Input: part model. Units: mm. Frame: model coordinates. A direction names the side the tool comes from. Round coordinates to 2 decimals unless told otherwise and drop trailing zeros. Loops run counter-clockwise (first coordinate to the right, second up) from the corner with the lowest first, then second, coordinate; pieces in that order, holes last. Notation, with made-up numbers: (77.25, 69.5) -> (85.25, 69.5) arc R29 ccw to (85.25, 89.5) -> close; hole circle Ø10 at (25.5, -8.5). An arc over 180 degrees is marked (long way). Answer as a JSON object with one key per item and string values. Group by question number.
Item 1: Material intervals for line 1 (Y direction, x = 60, z = 59.5); line 2 (X direction, y = 62, z = 2); line 3 (Z direction, x = 28.5, y = 12.5), sorted ascending. Write a range as [from, to].
Item 2: Section query A-A on x = 0. Return loops of the section in (y, z).
Item 3: Draft query along Y for faces 1 (the flat face through (75.115, 1, -4)), 2 (the flat face through (-65, 71.785, 51)), 3 (the flat face through (65, -60.993, 51)). Return one class per face: released by +Y, released by -Y, zero draft, split by the parting line, or undercut.
Item 4: Section query D-D on x = 63.5. Return loops of the section in (y, z).
Item 5: Set-up query: faces 4 (the flat face through (-65, -71.785, 51)), 5 (the flat face through (70.377, 66, 51)), 6 (the flat face through (-59.117, -66, 51)), 7 (the flat face through (-70.377, -66, 51)), 8 (the cylindrical face through (-0.47, 21.17, -4.44)). Return all of +Z, -Z, +X, -X, +Y, -Y with unobstructed straight access to the full face (end or side cutting, diameter ignored); none if empty.
Item 6: Section query C-C on y = 17. Return loops of the section in (x, z), and give its area (3 significant figures).
Item 7: Section query B-B on z = 69. Return loops of the section in (x, y), and give its area (3 significant figures).
Item 8: Pin query (flat end, axial travel): pin 1 (12 mm diameter, centred on y = -68, z = 36, fed in from +X); pin 2 (8.5 mm diameter, centred on y = 65, z = 37, fed in from -X); pin 3 (2 mm diameter, centred on y = -58, z = 59, fed in from +X); pin 4 (5.5 mm diameter, centred on x = -66.5, z = 71.5, fed in from +Y). Return the tip coordinate at first contact, or that it passes through.
from build123d import *

# Parameters (mm, degrees)
F0_W     = 11.260315
F0_H     = 10.791138
F1_DEPTH = 104
F2_W     = 149.32213
F2_H     = 149.927892
F3_DEPTH = 9
F4_R     = 21.873079
F5_DEPTH = 9.001


with BuildPart() as f1:
    # F0 (on Top) → F1 (new body)
    with BuildSketch(Plane.XY):
        with Locations((-64.74682, -66.388942)):
            Rectangle(F0_W, F0_H)
    extrude(amount=F1_DEPTH)

    # F2 (on Top) → F3 (join)
    with BuildSketch(Plane.XY):
        with Locations((-0.454325, -0.151444)):
            Rectangle(F2_W, F2_H)
    extrude(amount=-F3_DEPTH)

    # F4 (on face) → F5 (cut, through all)
    with BuildSketch(Plane.XY):
        with Locations((0, 0.696229)):
            Circle(F4_R)
    extrude(amount=-F5_DEPTH, mode=Mode.SUBTRACT)

    # F6: F1 across plane


with BuildPart() as f1_1:
    add(f1.part)
    add(f1.part.mirror(Plane.XZ))

    # F7: F1 across plane


with BuildPart() as f1_2:
    add(f1_1.part)
    add(f1_1.part.mirror(Plane.YZ))


solid = f1_2.part
Solved:
{
 "1": {"line 1": "[-71.78, -60.99], [60.99, 71.78]", "line 2": "[-70.38, -59.12], [59.12, 70.38]", "line 3": "[-9, 0]"},
 "2": {"outline": "(-75.12, -9) -> (-21.18, -9) -> (-21.18, 0) -> (-75.12, 0) -> close; (21.18, -9) -> (75.12, -9) -> (75.12, 0) -> (21.18, 0) -> close"},
 "3": {"face 1": "zero draft", "face 2": "released by +Y", "face 3": "undercut"},
 "4": {"outline": "(-75.12, -9) -> (75.12, -9) -> (75.12, 0) -> (71.78, 0) -> (71.78, 104) -> (60.99, 104) -> (60.99, 0) -> (-60.99, 0) -> (-60.99, 104) -> (-71.78, 104) -> (-71.78, 0) -> (-75.12, 0) -> close"},
 "5": {"face 4": "+Z, +X, -X, -Y", "face 5": "+Z, +X, +Y, -Y", "face 6": "+Z, +Y, -Y", "face 7": "+Z, -X, +Y, -Y", "face 8": "+Z, -Z"},
 "6": {"outline": "(-75.12, -9) -> (-12.86, -9) -> (-12.86, 0) -> (-75.12, 0) -> close; (12.86, -9) -> (75.12, -9) -> (75.12, 0) -> (12.86, 0) -> close", "area": "1,120 mm²"},
 "7": {"outline": "(-70.38, -71.78) -> (-59.12, -71.78) -> (-59.12, -60.99) -> (-70.38, -60.99) -> close; (-70.38, 60.99) -> (-59.12, 60.99) -> (-59.12, 71.78) -> (-70.38, 71.78) -> close; (59.12, -71.78) -> (70.38, -71.78) -> (70.38, -60.99) -> (59.12, -60.99) -> close; (59.12, 60.99) -> (70.38, 60.99) -> (70.38, 71.78) -> (59.12, 71.78) -> close", "area": "486 mm²"},
 "8": {"pin 1": "x = 70.38", "pin 2": "x = -70.38", "pin 3": "through", "pin 4": "y = 71.78"}
}
